Read the model definition and answer for the solid it produces. Units are mm, in the model's axes. A direction names the side the tool comes from. Round coordinates to 2 decimals unless told otherwise and drop trailing zeros. Write each loop counter-clockwise with the first axis right and the second up, starting at its lowest first coordinate (ties: lowest second). Pieces come first, ordered by that corner, then holes. Notation, with made-up numbers: (-13.5, -34) - (36.5, -34) arc R36 cw to (36.5, 3) - close; hole circle Ø2 at (45.25, -16). An arc over 180 degrees is marked (long way). One line per item, written item: value. Start each with the question number.
(1) A cutting plane is placed at B-B, the plane z = 27.5. Determine the outline of the cut face in (x, y).
(2) Flat-ended cylindrical pins translate along their axes: pin 1 Ø0.9 at (x, y) = (-10, 1.5) entering from -Z; pin 2 Ø6 at (x, y) = (-13.5, 5.5) entering from +Z; pin 3 Ø2.5 at (y, z) = (1.5, 25) entering from +X; pin 4 Ø6 at (x, z) = (-29, 32) entering from +Y. Find the tip coordinate at first contact, or state that the pin passes through.
(3) Find the intervals of material crossed by L1, parallel to X at y = 2.5, z = 24.25; L2, parallel to X at y = 6, z = 31.5; L3, parallel to Y at x = -22, z = 19.75, in increasing order.
(4) A cutting plane is placed at D-D, the plane y = 4.25. Determine the outline of the cut face in (x, z).
(5) A cutting plane is placed at C-C, the plane y = 8.9. Determine the outline of the cut face in (x, z), plus the area to 3 significant figures.
(6) The mould has two halves that part along X. Classify faces 4 (the face through (-11, 1, 29.63)), 5 (the face through (-2.749, 8.994, 14.911)), 6 (the face through (1.73, 9, 26)): +X half, -X half, draft (parallel to the pull), parting line (faces both ways), or undercut.
(7) For faces 1 (the face through (-22, 3, 21)), 2 (the face through (0.21, 9.62, 23.24)), 3 (the face through (-32.77, 1, 25)), determine the directions among +Z, -Z, +X, -X, +Y, -Y from which every point of the face is accessible in a straight line to the end or side of a thin tool.
from build123d import *

# Parameters (mm, degrees)
SKETCH1_W           = 12.5
SKETCH1_H           = 2.5
SKETCH1_W_2         = 2.5
SKETCH1_H_2         = 12.5
SKETCH1_W_3         = 9
SKETCH1_H_3         = 6
BOSS_EXTRUDE1_DEPTH = 3
FILLET1_R           = 2
SKETCH1_4_W         = 3
SKETCH1_4_H         = 7.491405235
BOSS_EXTRUDE2_DEPTH = 11.4
SKETCH2_R           = 2.4
BOSS_EXTRUDE3_DEPTH = 3
FILLET2_R           = 8
SKETCH1_7_R         = 1.25
CUT_EXTRUDE2_DEPTH  = 54.067966791


with BuildPart() as part:
    # Sketch1 → Boss-Extrude1 (new body)
    with BuildSketch(Plane(origin=(0, 0, 0), x_dir=(1, 0, 0), z_dir=(0, 1, 0))):
        Polygon((-14.041444449, -20.12144272), (-14.041444449, -12.630037485), (-38.561763486, -12.630037485), (-38.561763486, -34.630037485), (-1.270220731, -34.630037485), (-1.270220731, -12.630037485), (-4.270220731, -12.630037485), (-4.270220731, -20.12144272), align=None)
        with Locations((-10.520220731, -30.880037485)):
            Rectangle(SKETCH1_W, SKETCH1_H, mode=Mode.SUBTRACT)
        with Locations((-34.020220731, -25.190037485)):
            Rectangle(SKETCH1_W_2, SKETCH1_H_2, mode=Mode.SUBTRACT)
        with Locations((-24.475907507, -25.190037485)):
            Rectangle(SKETCH1_W_3, SKETCH1_H_3, mode=Mode.SUBTRACT)
    extrude(amount=BOSS_EXTRUDE1_DEPTH)

    # Fillet1
    fillet1_edges = [part.edges().sort_by_distance(p)[0] for p in [
        (-14.041444449, 1.5, 20.12144272),
        (-4.270220731, 1.5, 20.12144272),
        (-1.270220731, 1.5, 34.630037485),
        (-38.561763486, 1.5, 34.630037485),
        (-38.561763486, 1.5, 12.630037485),
    ]]
    fillet(fillet1_edges, radius=FILLET1_R)

    # Sketch1_4 → Boss-Extrude2 (add)
    with BuildSketch(Plane(origin=(0, 0, 0), x_dir=(1, 0, 0), z_dir=(0, 1, 0))):
        with Locations((-2.770220731, -16.375740103)):
            Rectangle(SKETCH1_4_W, SKETCH1_4_H)
        Polygon((-4.270220731, -29.630037485), (-4.270220731, -32.130037485), (-4.270220731, -34.630037485), (-1.270220731, -34.630037485), (-1.270220731, -20.12144272), (-4.270220731, -20.12144272), align=None)
    extrude(amount=BOSS_EXTRUDE2_DEPTH)

    # Sketch2 → Boss-Extrude3 (add)
    with BuildSketch(Plane(origin=(-1.270220731, 0, 0), x_dir=(0, 0, -1), z_dir=(1, 0, 0))):
        with Locations((-25.530037485, 8.9)):
            Circle(SKETCH2_R)
    extrude(amount=BOSS_EXTRUDE3_DEPTH)

    # Fillet2
    fillet2_edges = [part.edges().sort_by_distance(p)[0] for p in [
        (-2.770220731, 11.4, 12.630037485),
        (-2.770220731, 11.4, 34.630037485),
    ]]
    fillet(fillet2_edges, radius=FILLET2_R)

    # Sketch1_7 → Cut-Extrude2 (cut, through all)
    with BuildSketch(Plane(origin=(0, 0, 0), x_dir=(1, 0, 0), z_dir=(0, 1, 0))):
        with Locations(Location((-19.270220731, -32.130037485, 0), (0, 0, 270))):
            Circle(SKETCH1_7_R)
        with Locations(Location((-19.270220731, -15.130037485, 0), (0, 0, 270))):
            Circle(SKETCH1_7_R)
    extrude(amount=CUT_EXTRUDE2_DEPTH, mode=Mode.SUBTRACT)


solid = part.part
Here are the results:
1. outline: (-38.56, 0) - (-35.27, 0) - (-35.27, 3) - (-38.56, 3) - close; (-32.77, 0) - (-28.98, 0) - (-28.98, 3) - (-32.77, 3) - close; (-19.98, 0) - (-1.27, 0) - (-1.27, 7.53) - (1.73, 7.53) - (1.73, 10.27) - (-1.27, 10.27) - (-1.27, 11.35) - (-4.27, 11.35) - (-4.27, 3) - (-19.98, 3) - close
2. pin 1: z = 20.12
2. pin 2: z = 34.63
2. pin 3: x = -1.27
2. pin 4: y = 3
3. L1: -38.56 to -35.27, -32.77 to -28.98, -19.98 to -1.27
3. L2: -4.27 to -1.27
3. L3: 0 to 3
4. outline: (-4.27, 12.68) - (-1.27, 12.68) - (-1.27, 34.58) - (-4.27, 34.58) - close
5. outline: (-4.27, 14.82) - (-1.27, 14.82) - (-1.27, 23.13) - (1.73, 23.13) - (1.73, 27.93) - (-1.27, 27.93) - (-1.27, 32.44) - (-4.27, 32.44) - close
5. area: 67.3 mm²
6. face 4: undercut
6. face 5: draft
6. face 6: +X half
7. face 1: +Z, -Z, -X, +Y
7. face 2: +X
7. face 3: +Y, -Y
